from build123d import *

# Parameters (mm, degrees)
EXTRUDE_1_DEPTH               = 400
HOLE_WIZARD_M51_AT_2_COUNT    = 2
HOLE_WIZARD_M51_AT_2_PITCH    = 60
HOLE_WIZARD_M51_AT_3_COUNT    = 2
HOLE_WIZARD_M51_AT_3_PITCH    = 69.971422738
HOLE_WIZARD_M51_AT_4_COUNT    = 2
HOLE_WIZARD_M51_AT_4_PITCH    = 36
HOLE_WIZARD_M51_AT_5_COUNT    = 2
HOLE_WIZARD_M51_AT_5_PITCH    = 350
HOLE_WIZARD_M51_AT_6_COUNT    = 2
HOLE_WIZARD_M51_AT_6_PITCH    = 355.105618091
HOLE_WIZARD_M51_AT_7_COUNT    = 2
HOLE_WIZARD_M51_AT_7_PITCH    = 390.635379862
HOLE_WIZARD_M51_AT_8_COUNT    = 2
HOLE_WIZARD_M51_AT_8_PITCH    = 386
HOLE_WIZARD_M41_D             = 3.3
HOLE_WIZARD_M41_DEPTH         = 11.5
HOLE_WIZARD_M41_CSINK_D       = 4.05
HOLE_WIZARD_M41_CSINK_ANGLE   = 120
HOLE_WIZARD_M41_TIP           = 0.991420021
HOLE_WIZARD_M42_D             = 3.3
HOLE_WIZARD_M42_DEPTH         = 11.5
HOLE_WIZARD_M42_CSINK_D       = 4.05
HOLE_WIZARD_M42_CSINK_ANGLE   = 120
HOLE_WIZARD_M42_TIP           = 0.991420021
SKETCH_8_R                    = 14
CUT_EXTRUDE_2_DEPTH           = 10
EXTRUDE_2_DEPTH               = 10
CUT_EXTRUDE_3_DEPTH           = 425.970587218
SKETCH_12_W                   = 100
SKETCH_12_H                   = 5
EXTRUDE_3_DEPTH               = 20
HOLE_WIZARD_M41_2_D           = 4.5
HOLE_WIZARD_M41_2_DEPTH       = 5
HOLE_WIZARD_M41_2_CSINK_D     = 9.18
HOLE_WIZARD_M41_2_CSINK_ANGLE = 90


with BuildPart() as part:
    # Эскиз1 → Бобышка-Вытянуть1 (new body)
    with BuildSketch(Plane.XY):
        Polygon((0, 0), (0, 50), (5, 50), (5, 5), (95, 5), (95, 50), (100, 50), (100, 0), align=None)
    extrude(amount=EXTRUDE_1_DEPTH)

    # Эскиз9 → Зенковка для винта с потайной головкой и внутренним шестигранником M51 (revolve, cut)
    with BuildSketch(Plane(origin=(80, 5, 393), x_dir=(0, 0, 1), z_dir=(1, 0, 0))):
        Polygon((0, 0), (0, 5), (2.75, 5), (2.75, 2.985), (5.735, 0), align=None)
    hole_wizard_m51 = revolve(axis=Axis((80, 11.35, 393), (0, -1, 0)), mode=Mode.SUBTRACT)

    # Зенковка для винта с потайной головкой и внутренним шестигранником M51 at 2: Зенковка для винта с потайной головкой и внутренним шестигранником M51 ×2
    with Locations(*[(-i * HOLE_WIZARD_M51_AT_2_PITCH, 0, 0) for i in range(1, HOLE_WIZARD_M51_AT_2_COUNT)]):
        add(hole_wizard_m51, mode=Mode.SUBTRACT)

    # Зенковка для винта с потайной головкой и внутренним шестигранником M51 at 3: Зенковка для винта с потайной головкой и внутренним шестигранником M51 ×2
    with Locations(*[Vector(-0.8574929257125445, 0, -0.514495755427526) * (i * HOLE_WIZARD_M51_AT_3_PITCH) for i in range(1, HOLE_WIZARD_M51_AT_3_COUNT)]):
        add(hole_wizard_m51, mode=Mode.SUBTRACT)

    # Зенковка для винта с потайной головкой и внутренним шестигранником M51 at 4: Зенковка для винта с потайной головкой и внутренним шестигранником M51 ×2
    with Locations(*[(0, 0, -i * HOLE_WIZARD_M51_AT_4_PITCH) for i in range(1, HOLE_WIZARD_M51_AT_4_COUNT)]):
        add(hole_wizard_m51, mode=Mode.SUBTRACT)

    # Зенковка для винта с потайной головкой и внутренним шестигранником M51 at 5: Зенковка для винта с потайной головкой и внутренним шестигранником M51 ×2
    with Locations(*[(0, 0, -i * HOLE_WIZARD_M51_AT_5_PITCH) for i in range(1, HOLE_WIZARD_M51_AT_5_COUNT)]):
        add(hole_wizard_m51, mode=Mode.SUBTRACT)

    # Зенковка для винта с потайной головкой и внутренним шестигранником M51 at 6: Зенковка для винта с потайной головкой и внутренним шестигранником M51 ×2
    with Locations(*[Vector(-0.16896381511084574, 0, -0.9856222548132667) * (i * HOLE_WIZARD_M51_AT_6_PITCH) for i in range(1, HOLE_WIZARD_M51_AT_6_COUNT)]):
        add(hole_wizard_m51, mode=Mode.SUBTRACT)

    # Зенковка для винта с потайной головкой и внутренним шестигранником M51 at 7: Зенковка для винта с потайной головкой и внутренним шестигранником M51 ×2
    with Locations(*[Vector(-0.1535959185806014, 0, -0.9881337428685356) * (i * HOLE_WIZARD_M51_AT_7_PITCH) for i in range(1, HOLE_WIZARD_M51_AT_7_COUNT)]):
        add(hole_wizard_m51, mode=Mode.SUBTRACT)

    # Зенковка для винта с потайной головкой и внутренним шестигранником M51 at 8: Зенковка для винта с потайной головкой и внутренним шестигранником M51 ×2
    with Locations(*[(0, 0, -i * HOLE_WIZARD_M51_AT_8_PITCH) for i in range(1, HOLE_WIZARD_M51_AT_8_COUNT)]):
        add(hole_wizard_m51, mode=Mode.SUBTRACT)

    # Hole Wizard M41
    with Locations(Plane.ZY):
        with Locations((84, 12), (316, 12)):
            CounterSinkHole(HOLE_WIZARD_M41_D / 2, HOLE_WIZARD_M41_CSINK_D / 2, depth=HOLE_WIZARD_M41_DEPTH, counter_sink_angle=HOLE_WIZARD_M41_CSINK_ANGLE)
            with Locations((0, 0, -(HOLE_WIZARD_M41_DEPTH + HOLE_WIZARD_M41_TIP / 2))):  # 118° drill point
                Cone(0, HOLE_WIZARD_M41_D / 2, HOLE_WIZARD_M41_TIP, mode=Mode.SUBTRACT)

    # Отверстие обработанное метчиком M42
    with Locations(Plane.ZY):
        with Locations((320.5, 35), (320.5, 45), (79.5, 45), (79.5, 35)):
            CounterSinkHole(HOLE_WIZARD_M42_D / 2, HOLE_WIZARD_M42_CSINK_D / 2, depth=HOLE_WIZARD_M42_DEPTH, counter_sink_angle=HOLE_WIZARD_M42_CSINK_ANGLE)
            with Locations((0, 0, -(HOLE_WIZARD_M42_DEPTH + HOLE_WIZARD_M42_TIP / 2))):  # 118° drill point
                Cone(0, HOLE_WIZARD_M42_D / 2, HOLE_WIZARD_M42_TIP, mode=Mode.SUBTRACT)

    # Эскиз8 → Вырез-Вытянуть2 (cut)
    with BuildSketch(Plane(origin=(5, 0, 0), x_dir=(0, 0, -1), z_dir=(1, 0, 0))):
        with Locations((-340, 19)):
            Circle(SKETCH_8_R)
        with Locations((-60, 19)):
            Circle(SKETCH_8_R)
    extrude(amount=-CUT_EXTRUDE_2_DEPTH, mode=Mode.SUBTRACT)

    # Эскиз3 → Бобышка-Вытянуть2 (add)
    with BuildSketch(Plane.XY.offset(400)):
        Polygon((95, 5), (5, 5), (5, 50), (0, 50), (0, 0), (100, 0), (100, 50), (95, 50), align=None)
    extrude(amount=EXTRUDE_2_DEPTH)

    # Эскиз11 → Вырез-Вытянуть3 (cut, through all)
    with BuildSketch(Plane(origin=(100, 0, 0), x_dir=(0, 0, -1), z_dir=(1, 0, 0))):
        Polygon((-410, 10), (-410, 5), (-410, 0), (-405, 0), (-405, 5), (-388, 5), (-388, 10), (-378, 50), (-410, 50), align=None)
        Polygon((0, 5), (-10, 5), (-20, 50), (0, 50), align=None)
    extrude(amount=-CUT_EXTRUDE_3_DEPTH, mode=Mode.SUBTRACT)

    # Эскиз12 → Бобышка-Вытянуть3 (add)
    with BuildSketch(Plane(origin=(0, 0, 0), x_dir=(-1, 0, 0), z_dir=(0, 0, -1))):
        with Locations((-50, 2.5)):
            Rectangle(SKETCH_12_W, SKETCH_12_H)
    extrude(amount=EXTRUDE_3_DEPTH)

    # Hole Wizard M41 2
    with Locations(Plane(origin=(5, 0, 0), x_dir=(0, 0, -1), z_dir=(1, 0, 0))):
        with Locations((-365, 40), (-365, 15), (-35, 15), (-35, 40)):
            CounterSinkHole(HOLE_WIZARD_M41_2_D / 2, HOLE_WIZARD_M41_2_CSINK_D / 2, depth=HOLE_WIZARD_M41_2_DEPTH, counter_sink_angle=HOLE_WIZARD_M41_2_CSINK_ANGLE)


solid = part.part
Geometry: final body of the model. Coordinates: model frame, mm. A direction names the side the tool comes from. Give positions to 0.01 mm unless a question says otherwise; leave off trailing zeros. Order: outer loops, then holes, each group sorted by start corner. A loop starts at its lowest first (then second) coordinate and runs counter-clockwise, first axis right, second up. Notation, with made-up numbers: (-26.5, 76.5) -> (13.5, 76.5) arc R35 cw to (13.5, 115.5) -> close; hole circle Ø3 at (28.25, -27). An arc over 180 degrees is marked (long way). Write each question's results on one line, items separated by ' | '.
1) Cut plane A-A (z = 307.5). Output: boundary loops of the cut face in (x, y).
Geometry says:
outline: (0, 0) -> (100, 0) -> (100, 50) -> (95, 50) -> (95, 5) -> (5, 5) -> (5, 50) -> (0, 50) -> close
2) Cut plane B-B (x = 36). Output: boundary loops of the cut face in (y, z).
Geometry says:
outline: (0, -20) -> (5, -20) -> (5, 405) -> (0, 405) -> close
3) Line query: line 1 along X through (y, z) = (0.75, 43); line 2 along Z through (x, y) = (80, 1.25); line 3 along X through (y, z) = (44.5, 156). Output: solid intervals per line, ascending.
Geometry says:
line 1: x = 0 to 17.25, 22.75 to 77.25, 82.75 to 100 | line 2: z = -20 to 4.25, 9.75 to 40.25, 45.75 to 354.25, 359.75 to 390.25, 395.75 to 405 | line 3: x = 0 to 5, 95 to 100
4) First-contact query: pin 1 Ø3 at (x, z) = (45.5, 352.5) entering from +Y; pin 2 Ø1.5 at (x, y) = (16.5, 7.5) entering from +Z; pin 3 Ø6 at (y, z) = (14.5, 349.5) entering from -X; pin 4 Ø4 at (y, z) = (35, 320.5) entering from -X. Flat tips, straight axial feed; report the tip coordinate or a pass-through.
Geometry says:
pin 1: stops at y = 5 | pin 2: passes through | pin 3: stops at x = 95 | pin 4: stops at x = 0.01
5) Draft query along Y for faces 4 (the face through (2.77, 15.1, 362.64)), 5 (the face through (21.787, 2.202, 4.67)), 6 (the face through (95, 28, 196)). Return one class per face: released by +Y, released by -Y, zero draft, split by the parting line, or undercut.
Geometry says:
face 4: undercut | face 5: released by +Y | face 6: zero draft
6) Set-up query: faces 1 (the face through (2.535, 13.638, 327.068)), 2 (the face through (2.774, 13.562, 33.124)), 3 (the face through (5, 27, 196)). Return all of +Z, -Z, +X, -X, +Y, -Y with unobstructed straight access to the full face (end or side cutting, diameter ignored); none if empty.
Geometry says:
face 1: -X | face 2: none | face 3: +Z, -Z, +Y
